The figure shows three views and two pictorial views of one solid part (mm, origin at its lowest corner). Answer the questions. A direction names the side the tool comes from. Coordinates: 2 decimals unless noted, no trailing zeros. Loops run counter-clockwise (first coordinate to the right, second up) from the corner with the lowest first, then second, coordinate; pieces in that order, holes last. Notation, with made-up numbers: (-28.5, 56) - (21.5, 56) arc R32 ccw to (21.5, 87) - close; hole circle Ø2 at (3.5, 7). An arc over 180 degrees is marked (long way). Return JSON: item names as keys, results as strings. Group by question number.
1. Section A-A (x = 23) is taken. Write down the section's boundary in (y, z), and give its area (3 significant figures).
2. Section B-B (y = 16) is taken. Write down the section's boundary in (x, z).
3. The mould has two halves that part along X. Classify the marked faces 3, 4 and 5: pulls with the +X half, pulls with the -X half, needs draft (parallel to the pull), parting line crosses it, or undercut.
4. Section D-D (y = 25) is taken. Write down the section's boundary in (x, z).
5. Find the intervals of material crossed by line 1 along Y through (x, z) = (3.5, 2.6); line 2 along Y through (x, z) = (17, 2.15); line 3 along Y through (x, z) = (23, 2.85), in increasing order.
6. Which of the six approach directions +Z, -Z, +X, -X, +Y, -Y give full straight-line access (tool end or side, diameter ignored) to the marked faces 1 and 2?
7. Section C-C (x = 40.5) is taken. Write down the section's boundary in (y, z).
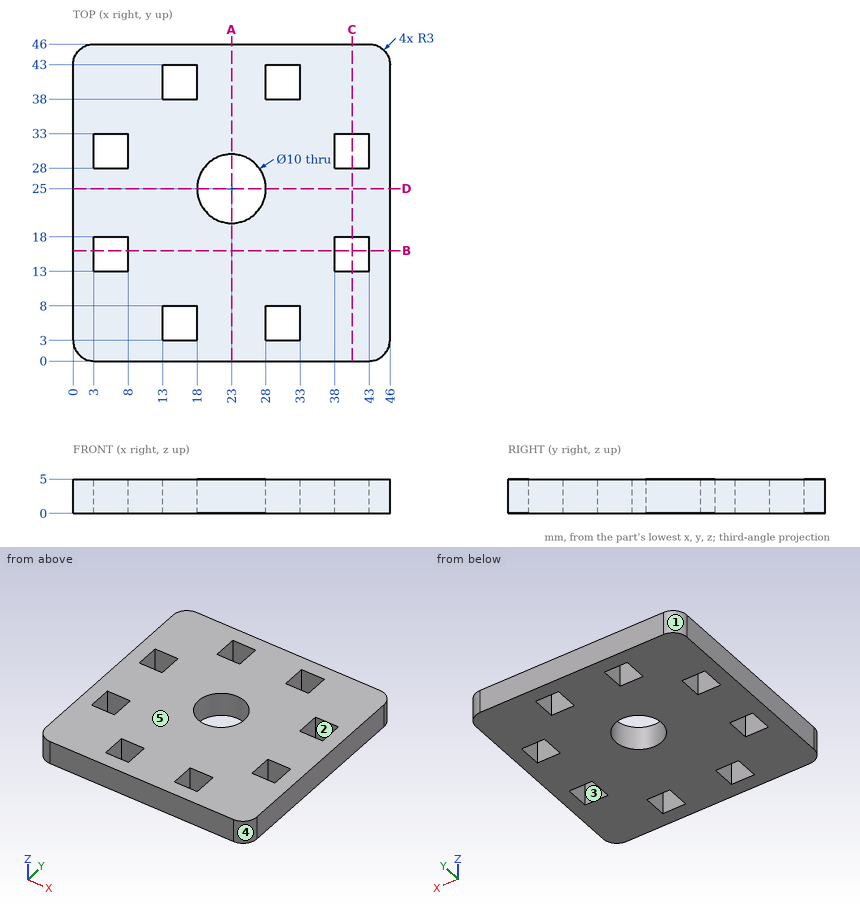
The answers:
{
 "1": {"outline": "(0, 0) - (20, 0) - (20, 5) - (0, 5) - close; (30, 0) - (46, 0) - (46, 5) - (30, 5) - close", "area": "180 mm2"},
 "2": {"outline": "(0, 0) - (3, 0) - (3, 5) - (0, 5) - close; (8, 0) - (38, 0) - (38, 5) - (8, 5) - close; (43, 0) - (46, 0) - (46, 5) - (43, 5) - close"},
 "3": {"face 3": "undercut", "face 4": "pulls with the +X half", "face 5": "needs draft"},
 "4": {"outline": "(0, 0) - (18, 0) - (18, 5) - (0, 5) - close; (28, 0) - (46, 0) - (46, 5) - (28, 5) - close"},
 "5": {"line 1": "y = 0 to 13, 18 to 28, 33 to 46", "line 2": "y = 0 to 3, 8 to 38, 43 to 46", "line 3": "y = 0 to 20, 30 to 46"},
 "6": {"face 1": "+Z, -Z, -X, +Y", "face 2": "+Z, -Z"},
 "7": {"outline": "(0, 0) - (13, 0) - (13, 5) - (0, 5) - close; (18, 0) - (28, 0) - (28, 5) - (18, 5) - close; (33, 0) - (46, 0) - (46, 5) - (33, 5) - close"}
}
